Design review of the part built by this model. Coordinates are the model's own, in mm. A direction names the side the tool comes from. Coordinates: 2 decimals unless noted, no trailing zeros. Loops run counter-clockwise (first coordinate to the right, second up) from the corner with the lowest first, then second, coordinate; pieces in that order, holes last. Notation, with made-up numbers: (-23, 77.5) -> (17, 77.5) arc R20 ccw to (17, 86.5) -> close; hole circle Ø9 at (-30, -14.5). An arc over 180 degrees is marked (long way). Use a Markdown table: item, result. Add a question column.
Q1. Take a section at D-D on x = -88. Write out the cut boundary in (y, z).
Q2. For faces 1 (the face through (-3, -53, 20)), 2 (the face through (-87.86, -81.75, 7.89)), 3 (the face through (-100, -87, 18)), 4 (the face through (-173, -49, -2)), 5 (the face through (-5, -5, 0)), list the 3-axis set-ups (+Z, -Z, +X, -X, +Y, -Y) from which the entire face can be reached by the end or side of a thin tool; tool diameter is ignored.
Q3. Take a section at C-C on y = -45.5. Count the separate pieces of the cut face and the enclosed holes in it, plus the area to 3 significant figures.
Q4. Draft analysis for pull direction Z (two halves, no side actions). For faces 6 (the face through (-173, -47, 13)), 7 (the face through (-134, -87, 16)), 8 (the face through (-172.14, -46.09, 18.1)), 9 (the face through (-8.935, -8.741, 7.888)), state which applies: pulls with the +Z half, pulls with the -Z half, needs draft (parallel to the pull), parting line crosses it, or undercut.
Q5. Clearance check with flat-ended pins moving along their axes: pin 1 Ø6.5 at (x, y) = (-4, -4.5) entering from -Z; pin 2 Ø2 at (x, y) = (-150, -86) entering from -Z; pin 3 Ø1.5 at (y, z) = (-85.5, 17) entering from +X. State where each tip first meets the part, or that it passes through.
Q6. For probe 1 along X at (y, z) = (-45.5, 20.55); probe 2 along Y at (x, z) = (-45.5, 20.5); probe 3 along Z at (x, y) = (-16, -8), list the stretches that pass through material, from the lowest coordinate up.
Q7. Take a section at A-A on z = 4. Write out the cut boundary in (x, y).
from build123d import *

# Parameters (mm, degrees)
SKETCH028_W          = 88
SKETCH028_H          = 3
PAD012_DEPTH         = 176
SKETCH029_R          = 25
POCKET015_DEPTH      = 100
POCKET015_DEPTH_BACK = 100
PAD014_DEPTH         = 19
SKETCH032_W          = 139
SKETCH032_H          = 6
SKETCH032_W_2        = 6
SKETCH032_H_2        = 69.5
POCKET016_DEPTH      = 20
SKETCH043_W          = 3
SKETCH043_H          = 88
PAD019_DEPTH         = 19
SKETCH044_W          = 3
SKETCH044_H          = 79
PAD020_DEPTH         = 6
PAD020_DEPTH_BACK    = 6
CHAMFER007_SIZE      = 2.99
CHAMFER008_SIZE      = 1.5
FILLET012_R          = 3
FILLET013_R          = 1
SKETCH086_W          = 67
SKETCH086_H          = 4.5
PAD037_DEPTH         = 3
CHAMFER011_SIZE      = 2.99
CHAMFER013_SIZE      = 1


with BuildPart() as part:
    # Sketch028 → Pad012 (new body)
    with BuildSketch(Plane.YZ):
        with Locations((-44, 20.5)):
            Rectangle(SKETCH028_W, SKETCH028_H)
    extrude(amount=-PAD012_DEPTH)

    # Sketch029 → Pocket015 (cut, two sides)
    with BuildSketch(Plane.XY) as pocket015_sk:
        with Locations((-130.5, -45.5)):
            Circle(SKETCH029_R)
        with Locations((-45.5, -45.5)):
            Circle(SKETCH029_R)
    extrude(amount=-POCKET015_DEPTH, mode=Mode.SUBTRACT)
    extrude(pocket015_sk.sketch, amount=POCKET015_DEPTH_BACK, mode=Mode.SUBTRACT)

    # Sketch031 → Pad014 (join)
    with BuildSketch(Plane.XY):
        with BuildLine():
            ThreePointArc((-12.5, 0), (-8.838835, -8.838835), (0, -12.5))
            Line((0, 0), (0, -12.5))
            Line((-12.5, 0), (0, 0))
        make_face()
        with BuildLine():
            ThreePointArc((-176, 0), (-169.75, -6.25), (-163.5, 0))
            Line((-176, 0), (-163.5, 0))
        make_face()
        with BuildLine():
            ThreePointArc((-81.75, -88), (-88, -81.75), (-94.25, -88))
            Line((-94.25, -88), (-81.75, -88))
        make_face()
    extrude(amount=PAD014_DEPTH)

    # Sketch032 → Pocket016 (cut)
    with BuildSketch(Plane.XY):
        with Locations((-88, -3)):
            Rectangle(SKETCH032_W, SKETCH032_H)
        with Locations((-3, -53.25)):
            Rectangle(SKETCH032_W_2, SKETCH032_H_2)
    extrude(amount=POCKET016_DEPTH, mode=Mode.SUBTRACT)

    # Sketch043 → Pad019 (join)
    with BuildSketch(Plane.XY):
        with Locations((-174.5, -44)):
            Rectangle(SKETCH043_W, SKETCH043_H)
    extrude(amount=PAD019_DEPTH)

    # Sketch044 → Pad020 (join, two sides)
    with BuildSketch(Plane.XY) as pad020_sk:
        with Locations((-171.5, -48.5)):
            Rectangle(SKETCH044_W, SKETCH044_H)
    extrude(amount=PAD020_DEPTH)
    extrude(pad020_sk.sketch, amount=-PAD020_DEPTH_BACK)

    # Chamfer007
    chamfer007_edges = [part.edges().sort_by_distance(p)[0] for p in [
        (-173, -48.5, 6),
    ]]
    chamfer(chamfer007_edges, length=CHAMFER007_SIZE)

    # Chamfer008
    chamfer008_edges = [part.edges().sort_by_distance(p)[0] for p in [
        (-173, -48.5, -6),
    ]]
    chamfer(chamfer008_edges, length=CHAMFER008_SIZE)

    # Fillet012
    fillet012_edges = [part.edges().sort_by_distance(p)[0] for p in [
        (-166.688138, -5.448624, 19),
        (-88, -81.75, 19),
        (-8.838835, -8.838835, 19),
        (-173, -46.66927, 19),
    ]]
    fillet(fillet012_edges, radius=FILLET012_R)

    # Fillet013
    fillet013_edges = [part.edges().sort_by_distance(p)[0] for p in [
        (-155.5, -45.5, 22),
        (-105.5, -45.5, 20.5),
        (-155.5, -45.5, 19),
        (-70.5, -45.5, 22),
        (-20.5, -45.5, 20.5),
        (-70.5, -45.5, 19),
        (-176, -44, 22),
    ]]
    fillet(fillet013_edges, radius=FILLET013_R)

    # Sketch086 → Pad037 (join)
    with BuildSketch(Plane.XY.offset(19)):
        with Locations((-133.5, -87.25)):
            Rectangle(SKETCH086_W, SKETCH086_H)
        with Locations((-42.5, -87.25)):
            Rectangle(SKETCH086_W, SKETCH086_H)
    extrude(amount=-PAD037_DEPTH)

    # Chamfer011
    chamfer011_edges = [part.edges().sort_by_distance(p)[0] for p in [
        (-133.5, -85, 19),
        (-42.5, -85, 19),
    ]]
    chamfer(chamfer011_edges, length=CHAMFER011_SIZE)

    # Chamfer013
    chamfer013_edges = [part.edges().sort_by_distance(p)[0] for p in [
        (-88, -88, 0),
    ]]
    chamfer(chamfer013_edges, length=CHAMFER013_SIZE)


solid = part.part
Answer list:
| question | item | result |
|---|---|---|
| 1 | outline | (-88, 1) -> (-87, 0) -> (-81.75, 0) -> (-81.75, 16) arc R3 cw to (-78.75, 19) -> (-6, 19) -> (-6, 20) -> (0, 20) -> (0, 22) -> (-88, 22) -> close |
| 2 | face 1 | -Z, +X, -Y |
| 2 | face 2 | -Z, +Y |
| 2 | face 3 | -Z, +Y, -Y |
| 2 | face 4 | -Z, -X, +Y, -Y |
| 2 | face 5 | -Z, +X, +Y, -Y |
| 3 | separate pieces | 3 |
| 3 | enclosed holes | 0 |
| 3 | area | 318 mm² |
| 4 | face 6 | undercut |
| 4 | face 7 | pulls with the -Z half |
| 4 | face 8 | undercut |
| 4 | face 9 | needs draft |
| 5 | pin 1 | z = 0 |
| 5 | pin 2 | z = 16 |
| 5 | pin 3 | x = -9 |
| 6 | probe 1 | -176 to -155.5, -105.5 to -70.5, -20.5 to 0 |
| 6 | probe 2 | -88 to -70.5, -20.5 to 0 |
| 6 | probe 3 | 19 to 22 |
| 7 | outline | (-176, -88) -> (-170, -88) -> (-170, -9) -> (-173, -9) -> (-173, -5.34) arc R6.25 ccw to (-163.5, 0) -> (-176, 0) -> close; (-94.25, -88) -> (-81.75, -88) arc R6.25 ccw to start; (-12.5, 0) arc R12.5 ccw to (0, -12.5) -> (0, 0) -> close |
